from build123d import *

# Parameters (mm, degrees)
BOSS_EXTRUDE1_DEPTH = 37
SKETCH4_W           = 8.655670696
SKETCH4_H           = 10.70324871
CUT_EXTRUDE1_DEPTH  = 2.886751346


with BuildPart() as part:
    # Sketch1 → Revolve1 (revolve)
    with BuildSketch(Plane.XY):
        Polygon((0, 2), (-4, 2), (-4, 0), (52.5, 0), (52.5, 1.5875), (46.5, 1.5875), (46.5, 2), (37, 2), (37, 2.5), (0, 2.5), align=None)
    revolve(axis=Axis((-6.185185185, 0, 0), (1, 0, 0)))

    # Sketch2 → Boss-Extrude1 (add)
    with BuildSketch(Plane(origin=(0, 0, 0), x_dir=(0, 0, -1), z_dir=(1, 0, 0))):
        Polygon((0, 2.886751346), (-2.5, 1.443375673), (-2.5, -1.443375673), (0, -2.886751346), (2.5, -1.443375673), (2.5, 1.443375673), align=None)
    extrude(amount=BOSS_EXTRUDE1_DEPTH)

    # Sketch4 → Cut-Extrude1 (cut, through all)
    with BuildSketch(Plane(origin=(0, 1, 0), x_dir=(1, 0, 0), z_dir=(0, 1, 0))):
        with Locations((51.827835348, -0.030836047)):
            Rectangle(SKETCH4_W, SKETCH4_H)
    extrude(amount=CUT_EXTRUDE1_DEPTH, mode=Mode.SUBTRACT)


solid = part.part
Check sheet for the modelled part. Datum: model origin and axes. Units: mm. A direction names the side the tool comes from. Give positions to 0.01 mm unless a question says otherwise; leave off trailing zeros. Order: outer loops, then holes, each group sorted by start corner. A loop starts at its lowest first (then second) coordinate and runs counter-clockwise, first axis right, second up. Notation, with made-up numbers: M 61.25,4.5 L 98.25,4.5 A14 ccw 98.25,24.5 Z; hole C -32,50.5 d5. An arc over 180 degrees is marked long. Answer as CSV lines item,"result". Start each with the question number.
Item 1: Cross-section at C-C on z = -0.75. Enter the section's corners in (x, y).
Item 2: Thickness scan on line 1 (X direction, y = 0.65, z = 2); line 2 (X direction, y = 1.25, z = 0.4); line 3 (Y direction, x = 23.5, z = 1.35). Record the ranges inside material, lowest first. Write a range as [from, to].
Item 3: Gauge pin test, flat ends, axial feed: P1, Ø2.5, axis at x = 51, z = 0, coming from the +Y side; P2, Ø1, axis at x = 27, z = -1, coming from the -Y side. Record the tip position at first contact, or that the pin passes through.
Item 4: Cross-section at B-B on x = 16.5. Enter the section's corners in (y, z).
Item 5: Tool access check on faces 1 (the face through (-2, 0, -2)), 2 (the face through (50, 1, 0)), 3 (the face through (37, -2, 1)). Record the directions out of +Z, -Z, +X, -X, +Y, -Y that give a thin tool (end or side, any length) a straight path to the whole face; none if there is none.
Item 6: Cross-section at A-A on y = 0. Enter the section's corners in (x, z), plus the area to 3 significant figures.
Established:
1,outline,"M -4,-1.85 L 0,-1.85 L 0,-2.45 L 37,-2.45 L 37,-1.85 L 46.5,-1.85 L 46.5,-1.4 L 52.5,-1.4 L 52.5,1 L 47.5,1 L 47.5,1.4 L 46.5,1.4 L 46.5,1.85 L 37,1.85 L 37,2.45 L 0,2.45 L 0,1.85 L -4,1.85 Z"
2,line 1,"x = [0, 37]"
2,line 2,"x = [-4, 47.5]"
2,line 3,"y = [-2.11, 2.11]"
3,P1,"stops at y = 1"
3,P2,"stops at y = -2.6"
4,outline,"M -2.89,0 L -1.44,-2.5 L 1.44,-2.5 L 2.89,0 L 1.44,2.5 L -1.44,2.5 Z"
5,face 1,"-X"
5,face 2,"+Z, -Z, +X, +Y"
5,face 3,"+X"
6,outline,"M -4,-2 L 0,-2 L 0,-2.5 L 37,-2.5 L 37,-2 L 46.5,-2 L 46.5,-1.59 L 52.5,-1.59 L 52.5,1.59 L 46.5,1.59 L 46.5,2 L 37,2 L 37,2.5 L 0,2.5 L 0,2 L -4,2 Z"
6,area,"258 mm^2"
